from build123d import *

# Parameters (mm, degrees)
BOSS_EXTRUDE1_DEPTH         = 6.35
SKETCH3_R                   = 44.4881
SKETCH3_R_2                 = 12.7381
CUT_EXTRUDE1_DEPTH          = 7.35
F_1_4_CLEARANCE_HOLE1_D     = 6.7564
F_1_4_CLEARANCE_HOLE1_DEPTH = 25.4
F_1_4_CLEARANCE_HOLE1_TIP   = 2.029827343
SKETCH11_R                  = 44.4881
BOSS_EXTRUDE3_DEPTH         = 3.175
SKETCH12_R                  = 12.7381
BOSS_EXTRUDE4_DEPTH         = 3.175


with BuildPart() as part:
    # Sketch1 → Boss-Extrude1 (new body)
    with BuildSketch(Plane(origin=(0, 0, 0), x_dir=(1, 0, 0), z_dir=(0, 1, 0))):
        with BuildLine():
            Line((0, 53.3781), (49.391408666, 64.669508666))
            ThreePointArc((49.391408666, 64.669508666), (60.19465678, 60.19465678), (64.669508666, 49.391408666))
            Line((64.669508666, 49.391408666), (53.3781, 0))
            ThreePointArc((53.3781, 0), (-37.744016477, -37.744016477), (0, 53.3781))
        make_face()
    extrude(amount=BOSS_EXTRUDE1_DEPTH)

    # Sketch3 → Cut-Extrude1 (cut, through all)
    with BuildSketch(Plane(origin=(0, 6.35, 0), x_dir=(1, 0, 0), z_dir=(0, 1, 0))):
        Circle(SKETCH3_R)
        with Locations((49.391408666, 49.391408666)):
            Circle(SKETCH3_R_2)
    extrude(amount=-CUT_EXTRUDE1_DEPTH, mode=Mode.SUBTRACT)

    # 1/4 Clearance Hole1
    with Locations(Plane.XZ):
        with Locations((49.391408666, -17.641408666), (17.641408666, -49.391408666)):
            Hole(F_1_4_CLEARANCE_HOLE1_D / 2, depth=F_1_4_CLEARANCE_HOLE1_DEPTH)
            with Locations((0, 0, -(F_1_4_CLEARANCE_HOLE1_DEPTH + F_1_4_CLEARANCE_HOLE1_TIP / 2))):  # 118° drill point
                Cone(0, F_1_4_CLEARANCE_HOLE1_D / 2, F_1_4_CLEARANCE_HOLE1_TIP, mode=Mode.SUBTRACT)

    # Sketch11 → Boss-Extrude3 (add)
    with BuildSketch(Plane(origin=(0, 6.35, 0), x_dir=(-1, 0, 0), z_dir=(0, 1, 0))):
        Circle(SKETCH11_R)
    extrude(amount=-BOSS_EXTRUDE3_DEPTH)

    # Sketch12 → Boss-Extrude4 (add)
    with BuildSketch(Plane(origin=(0, 6.35, 0), x_dir=(-1, 0, 0), z_dir=(0, 1, 0))):
        with Locations((-49.391408666, -49.391408666)):
            Circle(SKETCH12_R)
    extrude(amount=-BOSS_EXTRUDE4_DEPTH)


solid = part.part
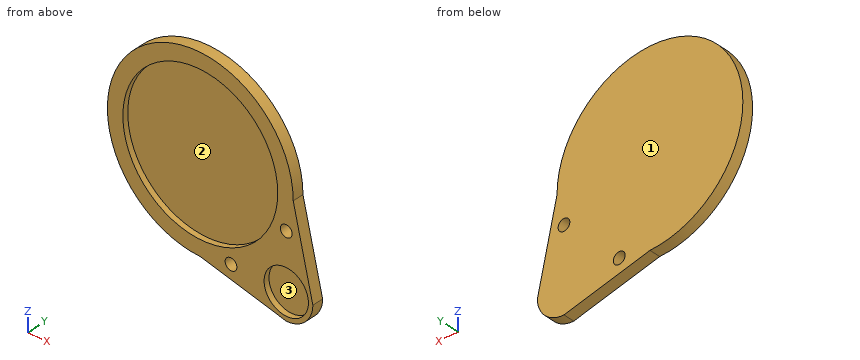
CAD build for the part. Positions are in the model's coordinates, mm. Face numbers are marked on the shaded views. Give positions to 0.01 mm unless a question says otherwise; leave off trailing zeros. Order: outer loops, then holes, each group sorted by start corner. A loop starts at its lowest first (then second) coordinate and runs counter-clockwise, first axis right, second up. Notation, with made-up numbers: (-5.5, -22) - (46.5, -22) arc R35 ccw to (46.5, 12) - close; hole circle Ø3 at (27, 66). An arc over 180 degrees is marked (long way). Write each question's results on one line, items separated by ' | '.
1. Saw through at A-A on x = -42.5. List the corners of the cut face in (y, z) (3 decimals), and give its area (3 significant figures).
Calculated:
outline: (0, -32.295) - (6.35, -32.295) - (6.35, 32.295) - (0, 32.295) - (0, 13.151) - (3.175, 13.151) - (3.175, -13.151) - (0, -13.151) - close | area: 327 mm2
2. Pull direction Z, two halves, no side cores. Call the marked faces 1, 2 and 3: released by +Z, released by -Z, zero draft, split by the parting line, or undercut.
Calculated:
face 1: zero draft | face 2: undercut | face 3: undercut
3. Saw through at B-B on y = 5.25. List the corners of the cut face in (x, z), and give its area (3 significant figures).
Calculated:
outline: (0, -53.38) - (49.39, -64.67) arc R15.28 ccw to (64.67, -49.39) - (53.38, 0) arc R53.38 ccw (long way) to start; hole circle Ø6.76 at (17.64, -49.39); hole circle Ø6.76 at (49.39, -17.64) | area: 10,200 mm2
4. Pin check, flat tips, straight feed: pin 1 (12.5 mm diameter, centred on x = 44, z = -49.5, fed in from -Y) (3 decimals); pin 2 (2 mm diameter, centred on y = 2, z = -3, fed in from -X); pin 3 (1 mm diameter, centred on x = -35.5, y = 1, fed in from +Z); pin 4 (8 mm diameter, centred on x = 49.39, z = -17.64, fed in from +Y). Stop position of each tip, or through.
Calculated:
pin 1: stops at y = 3.175 | pin 2: stops at x = -53.34 | pin 3: stops at z = 40.3 | pin 4: stops at y = 6.35
5. Saw through at C-C on z = -29. List the corners of the cut face in (x, y) (3 decimals), and give its area (3 significant figures).
Calculated:
outline: (-44.813, 0) - (-33.737, 0) - (-33.737, 3.175) - (33.737, 3.175) - (33.737, 0) - (60.008, 0) - (60.008, 6.35) - (-44.813, 6.35) - close | area: 451 mm2
6. Probe L1, parallel to Z at x = 0, y = 2.25; L2, parallel to X at y = 2.75, z = -15; L3, parallel to X at y = 2.5, z = 20.5. List the from-to ranges inside material, lowest first. Write a range as from..to.
Calculated:
L1: z = -53.38..-44.49, 44.49..53.38 | L2: x = -51.23..-41.88, 41.88..47.29, 51.5..56.81 | L3: x = -49.28..-39.48, 39.48..49.28
